Verification items for the finished model (mm, model axes). A direction names the side the tool comes from. Coordinates: 2 decimals unless noted, no trailing zeros. Write each loop counter-clockwise with the first axis right and the second up, starting at its lowest first coordinate (ties: lowest second). Pieces come first, ordered by that corner, then holes. Notation, with made-up numbers: (34.5, 85) -> (93.5, 85) arc R14 cw to (93.5, 105) -> close; hole circle Ø2 at (70.25, 54.5). An arc over 180 degrees is marked (long way). Answer in a Markdown table with one row per item.
```python
from build123d import *

# Parameters (mm, degrees)
F0_W     = 200
F0_H     = 200
F1_DEPTH = 10
F2_R     = 5
F3_R     = 5
F4_DEPTH = 25


with BuildPart() as f1:
    # F0 (on Front) → F1 (new body)
    with BuildSketch(Plane.XZ):
        Rectangle(F0_W, F0_H)
    extrude(amount=F1_DEPTH)

    # F2
    f2_edges = [f1.edges().sort_by_distance(p)[0] for p in [
        (-100, -5, 100),
        (-100, -5, -100),
        (100, -5, -100),
        (100, -5, 100),
    ]]
    fillet(f2_edges, radius=F2_R)

    # F3 (on face) → F4 (join)
    with BuildSketch(Plane.XZ.offset(10)):
        with Locations((-61.405938, 40)):
            Circle(F3_R)
        with Locations((-26.405938, 40)):
            Circle(F3_R)
        with Locations((23.594062, 40)):
            Circle(F3_R)
        with Locations((20.524925, -30)):
            Circle(F3_R)
    extrude(amount=F4_DEPTH)


solid = f1.part
```
1. Tool access check on faces 1 (the cylindrical face through (-99, -5, -98)), 2 (the cylindrical face through (26.282, -22.325, 44.216)). Record the directions out of +Z, -Z, +X, -X, +Y, -Y that give a thin tool (end or side, any length) a straight path to the whole face; none if there is none.
Geometry says:
| item | result |
|---|---|
| face 1 | -Z, -X, +Y, -Y |
| face 2 | -Y |
2. Section check C-C, the plane x = 23. Record the boundary of the cut face in (y, z), plus the area to 3 significant figures.
Geometry says:
| item | result |
|---|---|
| outline | (-35, -34.34) -> (-10, -34.34) -> (-10, -100) -> (0, -100) -> (0, 100) -> (-10, 100) -> (-10, 44.96) -> (-35, 44.96) -> (-35, 35.04) -> (-10, 35.04) -> (-10, -25.66) -> (-35, -25.66) -> close |
| area | 2,470 mm^2 |
3. Section check A-A, the plane z = -30. Record the boundary of the cut face in (x, y).
Geometry says:
| item | result |
|---|---|
| outline | (-100, -10) -> (15.52, -10) -> (15.52, -35) -> (25.52, -35) -> (25.52, -10) -> (100, -10) -> (100, 0) -> (-100, 0) -> close |
4. Thickness scan on line 1 (X direction, y = -27.5, z = 44); line 2 (Y direction, x = -6.5, z = 42.5); line 3 (Z direction, x = 18, y = -29.5). Record the ranges inside material, lowest first. Write a range as from..to.
Geometry says:
| item | result |
|---|---|
| line 1 | -64.41..-58.41, -29.41..-23.41, 20.59..26.59 |
| line 2 | -10..0 |
| line 3 | -34.32..-25.68 |
5. Section check D-D, the plane z = 40. Record the boundary of the cut face in (x, y).
Geometry says:
| item | result |
|---|---|
| outline | (-100, -10) -> (-66.41, -10) -> (-66.41, -35) -> (-56.41, -35) -> (-56.41, -10) -> (-31.41, -10) -> (-31.41, -35) -> (-21.41, -35) -> (-21.41, -10) -> (18.59, -10) -> (18.59, -35) -> (28.59, -35) -> (28.59, -10) -> (100, -10) -> (100, 0) -> (-100, 0) -> close |
6. Section check B-B, the plane y = -13. Record the boundary of the cut face in (x, z), plus the area to 3 significant figures.
Geometry says:
| item | result |
|---|---|
| outline | circle Ø10 at (-61.41, 40); circle Ø10 at (-26.41, 40); circle Ø10 at (20.52, -30); circle Ø10 at (23.59, 40) |
| area | 314 mm^2 |
7. Depth check by flat-ended pin: P1, Ø10, axis at x = 44.5, z = -66, coming from the -Y side; P2, Ø8, axis at y = -20.5, z = -29, coming from the +X side. Enter the tip coordinate at first touch or a pass-through.
Geometry says:
| item | result |
|---|---|
| P1 | y = -10 |
| P2 | x = 25.52 |
8. Mould release check, pull along X, two halves, no side actions. Record for faces 3 (the cylindrical face through (98, -5, -99)), 4 (the flat face through (20, -35, -30)), 5 (the flat face through (-100, -5, -1)), 6 (the cylindrical face through (-62.057, -22.325, 44.957)): released by +X, released by -X, zero draft, split by the parting line, or undercut.
Geometry says:
| item | result |
|---|---|
| face 3 | released by +X |
| face 4 | zero draft |
| face 5 | released by -X |
| face 6 | undercut |
